Work out the finished part from the listing and answer in its coordinate system (mm). Face numbers are marked on the shaded views. A direction names the side the tool comes from. Round coordinates to 2 decimals unless told otherwise and drop trailing zeros. Write each loop counter-clockwise with the first axis right and the second up, starting at its lowest first coordinate (ties: lowest second). Pieces come first, ordered by that corner, then holes. Notation, with made-up numbers: M 52.25,74 L 83.25,74 A18 ccw 83.25,105 Z; hole C 35,-21.75 d8. An arc over 180 degrees is marked long. Answer in a Markdown table with one row per item.
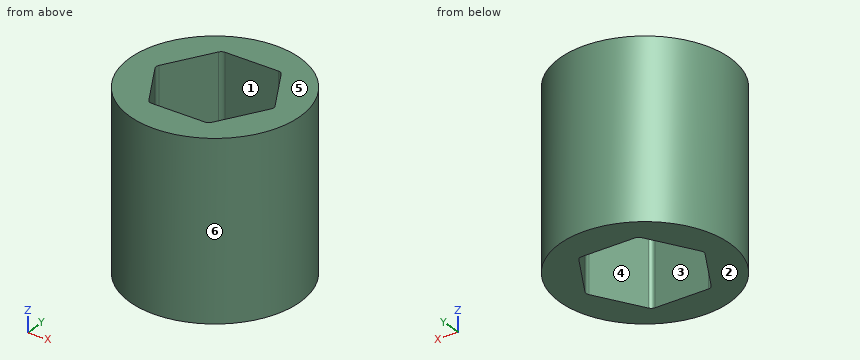
```python
from build123d import *

# Parameters (mm, degrees)
CROQUIS1_R              = 11.43
SALIENTE_EXTRUIR1_DEPTH = 11.764075024


with BuildPart() as part:
    # Croquis1 → Saliente-Extruir1 (new body, symmetric)
    with BuildSketch(Plane.XY):
        Circle(CROQUIS1_R)
        with BuildLine():
            Line((3.592850725, 6.985), (-3.592850725, 6.985))
            ThreePointArc((-3.592850725, 6.985), (-3.973850725, 6.882911358), (-4.252762083, 6.604))
            Line((-4.252762083, 6.604), (-7.845612808, 0.381))
            ThreePointArc((-7.845612808, 0.381), (-7.94770145, 0), (-7.845612808, -0.381))
            Line((-7.845612808, -0.381), (-4.252762083, -6.604))
            ThreePointArc((-4.252762083, -6.604), (-3.973850725, -6.882911358), (-3.592850725, -6.985))
            Line((-3.592850725, -6.985), (3.592850725, -6.985))
            ThreePointArc((3.592850725, -6.985), (3.973850725, -6.882911358), (4.252762083, -6.604))
            Line((4.252762083, -6.604), (7.845612808, -0.381))
            ThreePointArc((7.845612808, -0.381), (7.94770145, 0), (7.845612808, 0.381))
            Line((7.845612808, 0.381), (4.252762083, 6.604))
            ThreePointArc((4.252762083, 6.604), (3.973850725, 6.882911358), (3.592850725, 6.985))
        make_face(mode=Mode.SUBTRACT)
    extrude(amount=SALIENTE_EXTRUIR1_DEPTH, both=True)


solid = part.part
```
1. The part is cut by section C-C (y = 0). Determine the outline of the cut face in (x, z), plus the area to 3 significant figures.
Calculated:
| item | result |
|---|---|
| outline | M -11.43,-11.76 L -7.95,-11.76 L -7.95,11.76 L -11.43,11.76 Z; M 7.95,-11.76 L 11.43,-11.76 L 11.43,11.76 L 7.95,11.76 Z |
| area | 164 mm² |
2. The part is cut by section B-B (z = -9.75). Determine the outline of the cut face in (x, y) (3 decimals), plus the area to 3 significant figures.
Calculated:
| item | result |
|---|---|
| outline | C 0,0 d22.86; hole M -7.846,-0.381 L -4.253,-6.604 A0.762 ccw -3.593,-6.985 L 3.593,-6.985 A0.762 ccw 4.253,-6.604 L 7.846,-0.381 A0.762 ccw 7.846,0.381 L 4.253,6.604 A0.762 ccw 3.593,6.985 L -3.593,6.985 A0.762 ccw -4.253,6.604 L -7.846,0.381 A0.762 ccw Z |
| area | 242 mm² |
3. Consider line 1 along Y through (x, z) = (0, 2.5) (3 decimals); line 2 along X through (y, z) = (3, -4); line 3 along X through (y, z) = (3.25, -8.5). Determine where each line is inside the solid, lowest interval first. Write a range as from..to.
Calculated:
| item | result |
|---|---|
| line 1 | y = -11.43..-6.985, 6.985..11.43 |
| line 2 | x = -11.03..-6.33, 6.33..11.03 |
| line 3 | x = -10.96..-6.19, 6.19..10.96 |
4. Given pin 1 (1.5 mm diameter, centred on y = -4.5, z = 2, fed in from -X); pin 2 (3 mm diameter, centred on x = -3.5, z = 3.5, fed in from -Y); pin 3 (3 mm diameter, centred on y = 9, z = 9, fed in from +X), each flat-ended and moving along its own axis, determine where each tip first touches the part or whether it passes through.
Calculated:
| item | result |
|---|---|
| pin 1 | stops at x = -10.8 |
| pin 2 | stops at y = -11.25 |
| pin 3 | stops at x = 8.63 |
5. The part is cut by section D-D (x = 9.5). Determine the outline of the cut face in (y, z), plus the area to 3 significant figures.
Calculated:
| item | result |
|---|---|
| outline | M -6.36,-11.76 L 6.36,-11.76 L 6.36,11.76 L -6.36,11.76 Z |
| area | 299 mm² |
6. The part is cut by section A-A (x = 0). Determine the outline of the cut face in (y, z) (3 decimals), plus the area to 3 significant figures.
Calculated:
| item | result |
|---|---|
| outline | M -11.43,-11.764 L -6.985,-11.764 L -6.985,11.764 L -11.43,11.764 Z; M 6.985,-11.764 L 11.43,-11.764 L 11.43,11.764 L 6.985,11.764 Z |
| area | 209 mm² |
7. A tool of negligible diameter and unlimited length cuts with its end or side. For the marked faces 1 and 2, from which of +Z, -Z, +X, -X, +Y, -Y can it reach the whole face along a straight path? Write none if from no direction.
Calculated:
| item | result |
|---|---|
| face 1 | +Z, -Z |
| face 2 | -Z, +X, -X, +Y, -Y |
8. Determine the mould class of the marked faces 3, 4, 5 and 6 for opening direction X: released by +X, released by -X, zero draft, split by the parting line, or undercut.
Calculated:
| item | result |
|---|---|
| face 3 | undercut |
| face 4 | undercut |
| face 5 | zero draft |
| face 6 | split by the parting line |
